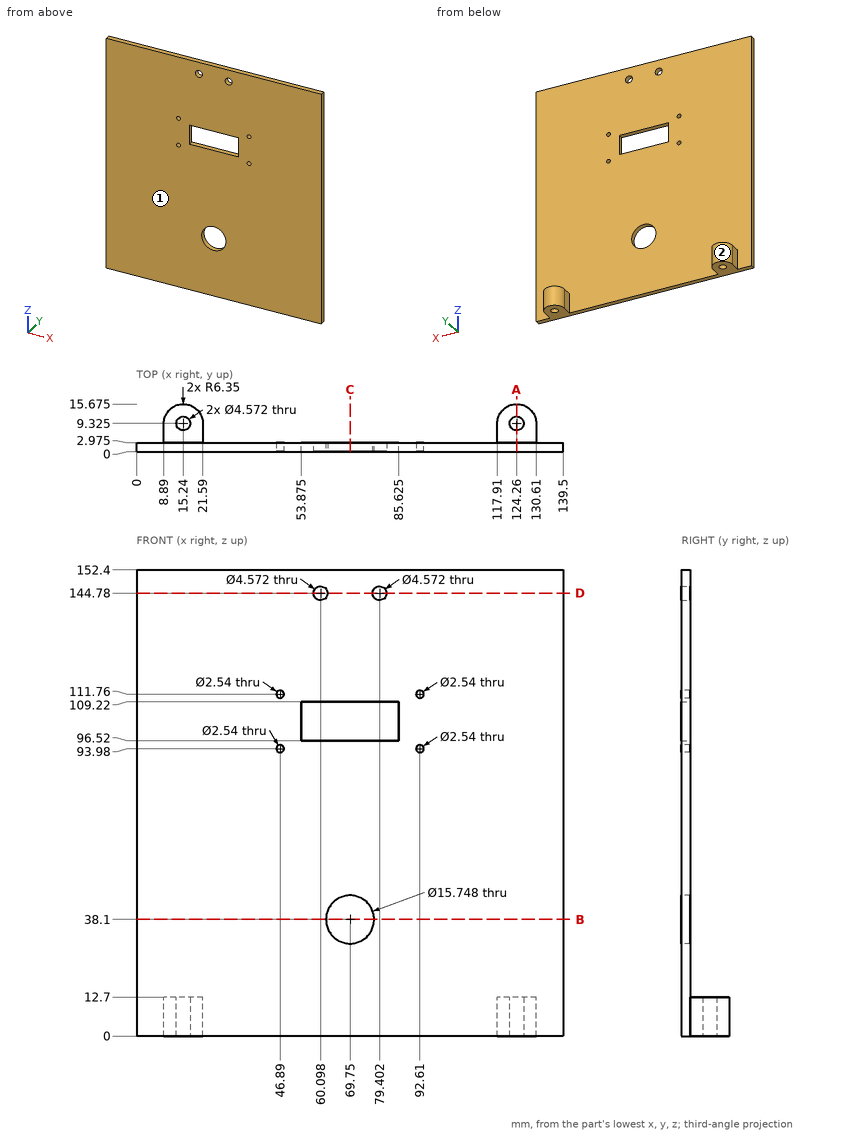
For this review, use the dimensioned drawing (mm, ordinates from the lowest corner) and the shaded views. Give positions to 0.01 mm unless a question says otherwise; leave off trailing zeros. Write each loop counter-clockwise with the first axis right and the second up, starting at its lowest first coordinate (ties: lowest second). Pieces come first, ordered by that corner, then holes. Notation, with made-up numbers: M 1.5,46 L 5.5,46 A22 cw 5.5,73 Z; hole C 22.25,50 d9. An arc over 180 degrees is marked long. Answer as a JSON object with one key per item and string values. Group by question number.
1) We need section D-D (z = 144.78). Give the boundary of the cut face in (x, y) (3 decimals).
2) We need section A-A (x = 124.26). Give the boundary of the cut face in (y, z) (3 decimals), and give its area (3 significant figures).
3) We need section C-C (x = 69.75). Give the boundary of the cut face in (y, z) (3 decimals), and give its area (3 significant figures).
4) We need section B-B (z = 38.1). Give the boundary of the cut face in (x, y) (3 decimals), and give its area (3 significant figures).
5) Clearance check with flat-ended pins moving along their axes: pin 1 Ø3 at (x, y) = (71.5, 5.5) entering from +Z; pin 2 Ø1.9 at (y, z) = (7, 3) entering from -X; pin 3 Ø4 at (x, z) = (119, 114.5) entering from +Y (3 decimals); pin 4 Ø1.9 at (y, z) = (4.5, 4.5) entering from +X. State where each tip first meets the part, or that it passes through.
6) For line 1 along Z through (x, y) = (46.89, 2); line 2 along X through (y, z) = (0.95, 93.98); line 3 along Y through (x, z) = (124, 6), list the stretches that pass through material, from the lowest coordinate up.
7) Mouldability with a two-part tool opening along X and no side actions: class the marked faces 1 and 2 as released by +X, released by -X, zero draft, split by the parting line, or undercut.
Answer key:
{
 "1": {"outline": "M 0,0 L 57.812,0 L 57.812,2.975 L 0,2.975 Z; M 62.384,0 L 77.116,0 L 77.116,2.975 L 62.384,2.975 Z; M 81.688,0 L 139.5,0 L 139.5,2.975 L 81.688,2.975 Z"},
 "2": {"outline": "M 0,0 L 7.039,0 L 7.039,12.7 L 2.975,12.7 L 2.975,152.4 L 0,152.4 Z; M 11.611,0 L 15.675,0 L 15.675,12.7 L 11.611,12.7 Z", "area": "557 mm²"},
 "3": {"outline": "M 0,0 L 2.975,0 L 2.975,30.226 L 0,30.226 Z; M 0,45.974 L 2.975,45.974 L 2.975,96.52 L 0,96.52 Z; M 0,109.22 L 2.975,109.22 L 2.975,152.4 L 0,152.4 Z", "area": "369 mm²"},
 "4": {"outline": "M 0,0 L 61.876,0 L 61.876,2.975 L 0,2.975 Z; M 77.624,0 L 139.5,0 L 139.5,2.975 L 77.624,2.975 Z", "area": "368 mm²"},
 "5": {"pin 1": "passes through", "pin 2": "stops at x = 8.89", "pin 3": "stops at y = 2.975", "pin 4": "stops at x = 130.61"},
 "6": {"line 1": "z = 0 to 92.71, 95.25 to 110.49, 113.03 to 152.4", "line 2": "x = 0 to 45.62, 48.16 to 91.34, 93.88 to 139.5", "line 3": "y = 0 to 7.05, 11.6 to 15.67"},
 "7": {"face 1": "zero draft", "face 2": "undercut"}
}
